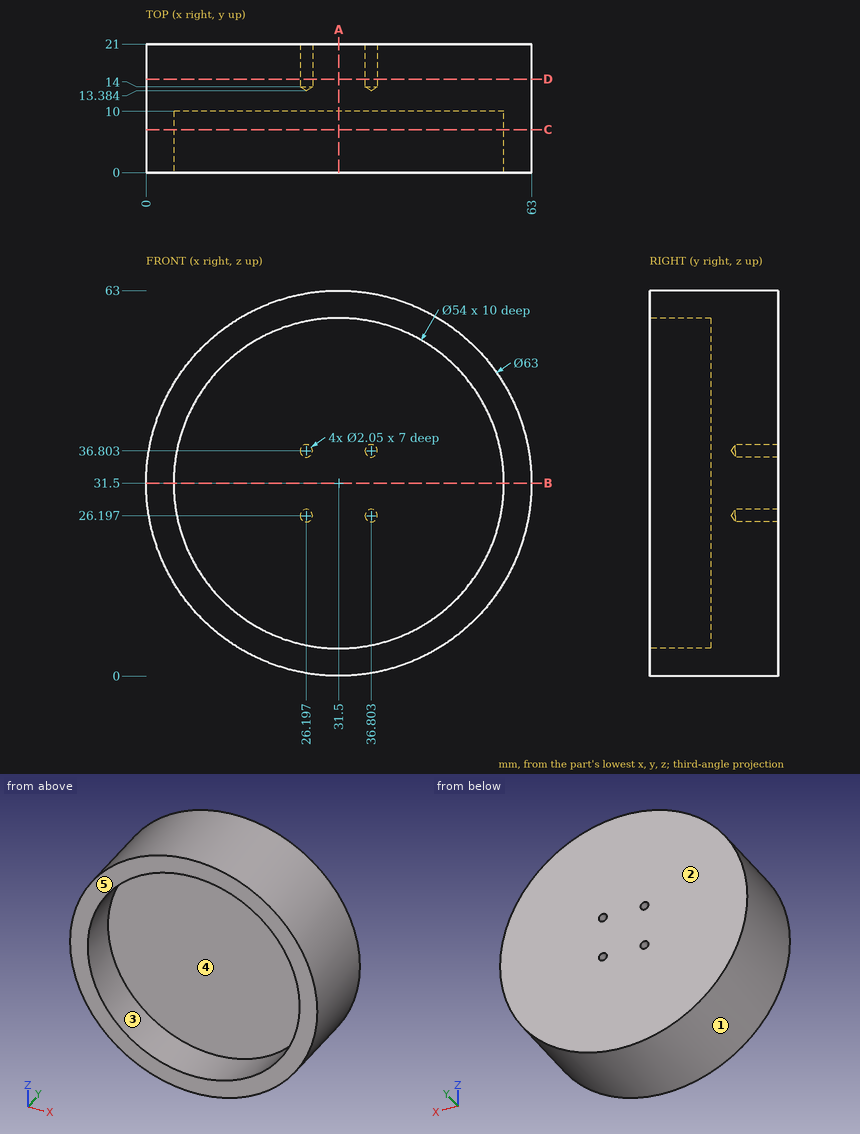
Print and shaded views of the part. All mm, measured from the part's lowest x, y and z. A direction names the side the tool comes from. Coordinates: 2 decimals unless noted, no trailing zeros. Order: outer loops, then holes, each group sorted by start corner. A loop starts at its lowest first (then second) coordinate and runs counter-clockwise, first axis right, second up.
(1) Slice it at A-A, the plane x = 31.5. Write the cut outline in (y, z).
Check sheet entries:
outline: (0, 0) - (21, 0) - (21, 63) - (0, 63) - (0, 58.5) - (10, 58.5) - (10, 4.5) - (0, 4.5) - close
(2) Pin check, flat tips, straight feed: pin 1 Ø1.5 at (x, y) = (52.5, 4.5) entering from +Z; pin 2 Ø1.8 at (x, z) = (36.8, 26.2) entering from -Y; pin 3 Ø2 at (y, z) = (11.5, 28) entering from -X. Stop position of each tip, or through.
Check sheet entries:
pin 1: stops at z = 55.63
pin 2: stops at y = 10
pin 3: stops at x = 0.1
(3) Slice it at B-B, the plane z = 31.5. Write the cut outline in (x, y), and give its area (3 significant figures).
Check sheet entries:
outline: (0, 0) - (4.5, 0) - (4.5, 10) - (58.5, 10) - (58.5, 0) - (63, 0) - (63, 21) - (0, 21) - close
area: 783 mm2
(4) Slice it at C-C, the plane y = 7. Write the cut outline in (x, z).
Check sheet entries:
outline: circle Ø63 at (31.5, 31.5); hole circle Ø54 at (31.5, 31.5)
(5) Probe L1, parallel to Z at x = 12, y = 7.75 (1 decimal); L2, parallel to Z at x = 43, y = 3.75 (1 decimal); L3, parallel to Y at x = 50, z = 17. List the from-to ranges inside material, lowest first.
Check sheet entries:
L1: z = 6.8 to 12.8, 50.2 to 56.2
L2: z = 2.2 to 7.1, 55.9 to 60.8
L3: y = 10 to 21
(6) Pull direction X, two halves, no side cores. Call the marked faces 1, 2 and 3: pulls with the +X half, pulls with the -X half, needs draft (parallel to the pull), parting line crosses it, or undercut.
Check sheet entries:
face 1: parting line crosses it
face 2: needs draft
face 3: undercut
(7) Slice it at D-D, the plane y = 15.25. State how many separate pieces and enclosed holes the cut face has, and give its area (3 significant figures).
Check sheet entries:
separate pieces: 1
enclosed holes: 4
area: 3,100 mm2
(8) Tool access for the marked faces 4 and 5: list every direction of +Z, -Z, +X, -X, +Y, -Y with a clear straight run to the whole face (end or side of a thin tool).
Check sheet entries:
face 4: -Y
face 5: +Z, -Z, +X, -X, -Y
